from build123d import *

# Parameters (mm, degrees)
F0_R          = 5.25
F1_DEPTH      = 5
F1_DEPTH_BACK = 5


with BuildPart() as f1:
    # F0 (on Front) → F1 (new body, two sides)
    with BuildSketch(Plane.XZ) as f1_sk:
        with BuildLine():
            ThreePointArc((11.5, 344.359994), (0, 355.859994), (-11.5, 344.359994))
            Line((-11.5, 344.359994), (-11.5, -55.640006))
            ThreePointArc((-11.5, -55.640006), (0, -67.140006), (11.5, -55.640006))
            Line((11.5, -55.640006), (11.5, 344.359994))
        make_face()
        with Locations((0, -56.160006)):
            Circle(F0_R, mode=Mode.SUBTRACT)
        with Locations((0, 344.359994)):
            Circle(F0_R, mode=Mode.SUBTRACT)
    extrude(amount=F1_DEPTH)
    extrude(f1_sk.sketch, amount=-F1_DEPTH_BACK)


solid = f1.part
Can you work these out from the model? Positions are in its coordinate system, mm. Coordinates: 2 decimals unless noted, no trailing zeros. Write each loop counter-clockwise with the first axis right and the second up, starting at its lowest first coordinate (ties: lowest second). Pieces come first, ordered by that corner, then holes. Notation, with made-up numbers: (-12.75, -22.5) -> (-2.75, -22.5) arc R22 cw to (-2.75, -10.5) -> close; hole circle Ø1 at (-34, -12). An arc over 180 degrees is marked (long way). Write each question's results on one line, items separated by ' | '. Start each with the question number.
Q1. We'd pull the mould along X, two halves only. Please class faces 1 (the face through (0, 5, 147)), 2 (the face through (-1.138, 0.07, 339.235)), 3 (the face through (0.253, -0.07, 355.857)), 4 (the face through (-1.138, 0.07, -61.285)): +X half, -X half, draft (parallel to the pull), parting line (faces both ways), or undercut.
Q2. I'm going to push flat-ended pins straight in: pin 1 (1.5 mm diameter, centred on x = -2, y = 3.5, fed in from +Z); pin 2 (12 mm diameter, centred on x = 0, z = -56.16, fed in from -Y). Where does each tip first touch, or does it pass through?
Q3. If I drill on probe 1 along Z at (x, y) = (0, 1.75); probe 2 along Z at (x, y) = (-3, -4.5); probe 3 along Z at (x, y) = (-9.5, -0.5), over which ranges is the centre line in solid material (lowest first)?
Q4. Imagine slicing it at B-B (y = -0.5). Write out the boundary of the cut face in (x, z), then the cut area to 3 significant figures.
Q5. Imagine slicing it at A-A (x = 0). Write out the boundary of the cut face in (y, z).
Taken from the geometry:
1) face 1: draft | face 2: undercut | face 3: parting line | face 4: undercut
2) pin 1: stops at z = 355.79 | pin 2: stops at y = -5
3) probe 1: z = -67.14 to -61.41, -50.91 to 339.11, 349.61 to 355.86 | probe 2: z = -66.74 to -60.47, -51.85 to 340.05, 348.67 to 355.46 | probe 3: z = -62.12 to 350.84
4) outline: (-11.5, -55.64) arc R11.5 ccw to (11.5, -55.64) -> (11.5, 344.36) arc R11.5 ccw to (-11.5, 344.36) -> close; hole circle Ø10.5 at (0, -56.16); hole circle Ø10.5 at (0, 344.36) | area: 9,440 mm^2
5) outline: (-5, -67.14) -> (5, -67.14) -> (5, -61.41) -> (-5, -61.41) -> close; (-5, -50.91) -> (5, -50.91) -> (5, 339.11) -> (-5, 339.11) -> close; (-5, 349.61) -> (5, 349.61) -> (5, 355.86) -> (-5, 355.86) -> close
